Design review of the part built by this model. Coordinates are the model's own, in mm. A direction names the side the tool comes from. Give positions to 0.01 mm unless a question says otherwise; leave off trailing zeros. Write each loop counter-clockwise with the first axis right and the second up, starting at its lowest first coordinate (ties: lowest second). Pieces come first, ordered by that corner, then holes. Notation, with made-up numbers: M 16,68.5 L 69,68.5 A26 ccw 69,92.5 Z; hole C 89.25,55.5 d7. An arc over 180 degrees is marked long. Write each question's results on one line, items separated by ' | '. Start each with the question number.
Autodesk Inventor part; units mm, degrees
ref_plane "YZ Plane" through (0, 0, 0) normal (1, 0, 0) x (0, 1, 0)
ref_plane "XZ Plane" through (0, 0, 0) normal (0, 1, 0) x (-1, 0, 0)
ref_plane "XY Plane" through (0, 0, 0) normal (0, 0, 1) x (1, 0, 0)
sketch "Sketch6" plane through (0, 0, 0) normal (1, 0, 0) x (0, 1, 0)
  line L0 (0, 0) -> (0, 100)
  line L1 (0, 100) -> (50, 100)
  line L2 (50, 100) -> (50, 95)
  line L3 (50, 95) -> (5, 95)
  line L4 (5, 95) -> (5, 5)
  line L5 (5, 5) -> (50, 5)
  line L6 (50, 5) -> (50, 0)
  line L7 (50, 0) -> (0, 0)
  line L8 (0, 100) -> (-14.5, 100)
  line L9 (-14.5, 100) -> (-14.5, 150)
  arc A0 (-14.5, 150) -> (25, 100) centre (36.8956, 150) ccw
  dimension "d66" = 14.5
  dimension "d67" = 50
  dimension "d68" = 50
  dimension "d69" = 45
  dimension "d87" = 90
extrude "Extrusion6" add sketch "Sketch6" along normal blind 200
sketch "Sketch7" plane through (0, 5, 95) normal (0, 0, -1) x (-1, 0, 0)
  line L0 (0, 45) -> (-200, 45)
  line L1 (0, 0) -> (-200, 0)
  line L2 (-200, 45) -> (-195, 45)
  line L3 (-195, 45) -> (-195, 0)
  line L4 (-195, 0) -> (-200, 0)
  line L5 (-200, 0) -> (-200, 45)
  point P0 (0, -5)
  dimension "d52" = 5
extrude "Extrusion7" add sketch "Sketch7" along normal blind 90
sketch "Sketch8" plane through (0, 5, 95) normal (0, 0, -1) x (-1, 0, 0)
  line L0 (0, 45) -> (-195, 45)
  line L1 (0, 0) -> (-195, 0)
  line L2 (0, 45) -> (-5, 45)
  line L3 (-5, 45) -> (-5, 0)
  line L4 (-5, 0) -> (0, 0)
  line L5 (0, 0) -> (0, 45)
  point P0 (0, -5)
  dimension "d55" = 5
extrude "Extrusion8" add sketch "Sketch8" along normal blind 90
sketch "Sketch9" plane through (200, 0, 0) normal (1, 0, 0) x (0, 0, -1)
  line L0 (0, 0) -> (0, 50)
  line L1 (-100, 0) -> (0, 0)
  line L2 (0, 50) -> (-75, 50)
  line L3 (-75, 50) -> (-75, 0)
  line L4 (-75, 0) -> (0, 0)
  line L5 (0, 0) -> (0, 50)
  circle A0 centre (-35, 18) radius 33.5
  dimension "d95" = 75
  dimension "d96" = 67
extrude "Extrusion9" cut sketch "Sketch9" against normal blind 35 contours L1 A0 L2 L0 | L1 A0 L2 | L1 L3 L2 A0
sketch "Sketch10" plane through (0, 0, 0) normal (-1, 0, 0) x (0, 0, 1)
  line L0 (0, 50) -> (100, 50)
  line L1 (100, 0) -> (0, 0)
  line L2 (0, 50) -> (75, 50)
  line L3 (75, 50) -> (75, 0)
  line L4 (75, 0) -> (0, 0)
  line L5 (0, 0) -> (0, 50)
  circle A0 centre (35, 18) radius 33.5
  dimension "d94" = 75
  dimension "d97" = 67
extrude "Extrusion10" cut sketch "Sketch10" against normal blind 35 contours L0 A0 L1 L5 | L0 A0 L1 | L0 L3 L1 A0
properties part number "intro 2 robot"
Q1. For faces 4 (the flat face through (99, 37, 100)), 5 (the flat face through (99, 0, 60)), 6 (the flat face through (35, 4.7, 23.4)), 7 (the flat face through (99, 27, 5)), 8 (the flat face through (5, 28, 85)), list the 3-axis set-ups (+Z, -Z, +X, -X, +Y, -Y) from which the entire face can be reached by the end or side of a thin tool; tool diameter is ignored.
Q2. We need section D-D on y = 16.5. Write out the cut boundary in (x, z), and give its area (3 significant figures).
Q3. For pin 1 Ø22.5 at (x, y) = (84.5, 25) entering from +Z; pin 2 Ø16 at (x, y) = (137, -8.5) entering from -Z; pin 3 Ø8 at (x, z) = (76, 29.5) entering from -Y; pin 4 Ø25 at (y, z) = (27.5, 36) entering from -X, all flat-tipped, find the tip position at first contact; note any pin that passes through.
Q4. We need section B-B on z = 88. Write out the cut boundary in (x, y), and give its area (3 significant figures).
Q5. The part is to be moulded in two halves that separate along X. For faces 1 (the flat face through (99, 5, 51)), 2 (the flat face through (0, 18, 96)), 3 (the flat face through (197, 16, 75)), say which applies: pulls with the +X half, pulls with the -X half, needs draft (parallel to the pull), parting line crosses it, or undercut.
Q6. We need section A-A on y = 28.5. Write out the cut boundary in (x, z), and give its area (3 significant figures).
Q7. Wall thickness on line 1 along X through (y, z) = (30, 82); line 2 along Z through (x, y) = (124, 39); line 3 along Y through (x, z) = (69, 57.5): over which ranges is each line inside the solid? List them lowest first. Write a range as from..to.
Q8. We need section C-C on x = 172. Write out the cut boundary in (y, z).
Answer sheet:
1) face 4: +Z, +X, -X, +Y | face 5: -Z, +X, -X, -Y | face 6: -Z, -X, +Y, -Y | face 7: +X, -X, +Y | face 8: -Z, +Y
2) outline: M 0,75 L 5,75 L 5,95 L 195,95 L 195,75 L 200,75 L 200,102.82 L 0,102.82 Z; M 35,0 L 165,0 L 165,5 L 35,5 Z | area: 2,410 mm^2
3) pin 1: z = 104.11 | pin 2: z = 100 | pin 3: y = 0 | pin 4: through
4) outline: M 0,0 L 200,0 L 200,50 L 195,50 L 195,5 L 5,5 L 5,50 L 0,50 Z | area: 1,450 mm^2
5) face 1: undercut | face 2: pulls with the -X half | face 3: needs draft
6) outline: M 0,75 L 5,75 L 5,95 L 195,95 L 195,75 L 200,75 L 200,100 L 0,100 Z; M 35,0 L 165,0 L 165,5 L 35,5 Z | area: 1,850 mm^2
7) line 1: 0..5, 195..200 | line 2: 0..5, 95..100 | line 3: 0..5
8) outline: M -14.5,100 L 0,100 L 0,75 L 5,75 L 5,95 L 50,95 L 50,100 L 25,100 A51.4 cw -14.5,150 Z
